Autodesk Inventor part; units mm, degrees
ref_plane "YZ Plane" through (0, 0, 0) normal (1, 0, 0) x (0, 1, 0)
ref_plane "XZ Plane" through (0, 0, 0) normal (0, 1, 0) x (-1, 0, 0)
ref_plane "XY Plane" through (0, 0, 0) normal (0, 0, 1) x (1, 0, 0)
sketch "Sketch1" plane through (0, 0, 0) normal (0, 1, 0) x (-1, 0, 0)
  line L0 (9, 9) -> (-9, 9)
  line L1 (-9, 9) -> (-9, -9)
  line L2 (-9, -9) -> (9, -9)
  line L3 (9, -9) -> (9, 9)
  line L4 (9, 9) -> (-9, -9) construction
  line L5 (-9, 9) -> (9, -9) construction
  line L6 (25, 10) -> (-25, 10)
  line L7 (-25, 10) -> (-25, -10)
  line L8 (-25, -10) -> (25, -10)
  line L9 (25, -10) -> (25, 10)
  line L10 (25, 10) -> (-25, -10) construction
  line L11 (-25, 10) -> (25, -10) construction
  line L12 (25, 0) -> (18, 0)
  line L13 (-25, 0) -> (-18, 0)
  circle A0 centre (18, 0) radius 2.5
  circle A1 centre (-18, 0) radius 2.5
  point P0 (0, 0)
  dimension "d0" = 18
  dimension "d1" = 18
  dimension "d2" = 50
  dimension "d3" = 20
  dimension "d4" = 7
  dimension "d5" = 5
  dimension "d6" = 5
extrude "Extrusion1" add sketch "Sketch1" along normal blind 3 contours L3 L2 L1 L0 | L9 L8 L7 L6
sketch "Sketch2" plane through (0, 3, 0) normal (0, 1, 0) x (1, 0, 0)
  line L0 (-9, 9) -> (9, 9)
  line L1 (9, 9) -> (9, -9)
  line L2 (9, -9) -> (-9, -9)
  line L3 (-9, -9) -> (-9, 9)
  line L4 (-9, 9) -> (9, -9) construction
  line L5 (9, 9) -> (-9, -9) construction
  circle A0 centre (-18, 0) radius 2.5
  circle A1 centre (18, 0) radius 2.5
  line L6 (-25, -10) -> (25, -10)
  line L7 (-25, 10) -> (25, 10)
  line L8 (25, 10) -> (25, -10)
  line L9 (25, -10) -> (-25, -10)
  line L10 (-25, -10) -> (-25, 10)
  line L11 (-25, 10) -> (25, -10) construction
  line L12 (25, 10) -> (-25, -10) construction
  point P0 (0, 0)
  dimension "d9" = 18
  dimension "d10" = 18
extrude "Extrusion2" add sketch "Sketch2" along normal blind 6
sketch "Sketch3" plane through (-25, 0, 10) normal (0, 0, 1) x (1, 0, 0)
  line L0 (34, 3) -> (34, 9)
  line L1 (16, -9) -> (34, -9)
  line L2 (34, -9) -> (34, 9)
  line L3 (34, 9) -> (16, 9)
  line L4 (16, 9) -> (16, -9)
  line L5 (16, -9) -> (34, 9) construction
  line L6 (34, -9) -> (16, 9) construction
  line L7 (16, 0) -> (34, 0)
  point P0 (25, 0)
extrude "Extrusion3" add sketch "Sketch3" along normal blind 10 contours L2 L7 L4 L3 L0
sketch "Sketch4" plane through (0, 9, 0) normal (0, 1, 0) x (1, 0, 0)
  line L0 (-9, -9) -> (9, -9)
  line L1 (0, -9) -> (0, -13)
  line L2 (4, -17) -> (-4, -17)
  line L3 (-4, -17) -> (-4, -9)
  line L4 (-4, -9) -> (4, -9)
  line L5 (4, -9) -> (4, -17)
  line L6 (4, -17) -> (-4, -9) construction
  line L7 (-4, -17) -> (4, -9) construction
  point P0 (0, 0)
  dimension "d15" = 4
  dimension "d16" = 8
extrude "Extrusion4" cut sketch "Sketch4" against normal blind 8
sketch "Sketch5" plane through (0, 3, 0) normal (0, 1, 0) x (1, 0, 0)
  line L0 (-4, -9) -> (4, -9)
  line L1 (0, -9) -> (0, -6)
  line L2 (0, -6) -> (-4, -6)
  line L3 (-4, -6) -> (-4, -9)
  line L4 (-4, -9) -> (0, -9)
  line L5 (0, -9) -> (0, -6)
  line L6 (0, -6) -> (4, -6)
  line L7 (4, -6) -> (4, -9)
  line L8 (4, -9) -> (0, -9)
  line L9 (0, -9) -> (0, -6)
  line L10 (-4, -6) -> (4, -6)
  line L11 (4, -6) -> (4, 0)
  line L12 (4, 0) -> (-4, 0)
  line L13 (-4, 0) -> (-4, -6)
  point P0 (0, 0)
  dimension "d19" = 3
extrude "Extrusion5" cut sketch "Sketch5" against normal blind 2
sketch "Sketch6" plane through (0, 3, 0) normal (0, 1, 0) x (1, 0, 0)
  circle A0 centre (0, 0) radius 2
  dimension "d22" = 4
extrude "Extrusion6" cut sketch "Sketch6" against normal through all
properties part number "gps_holder"
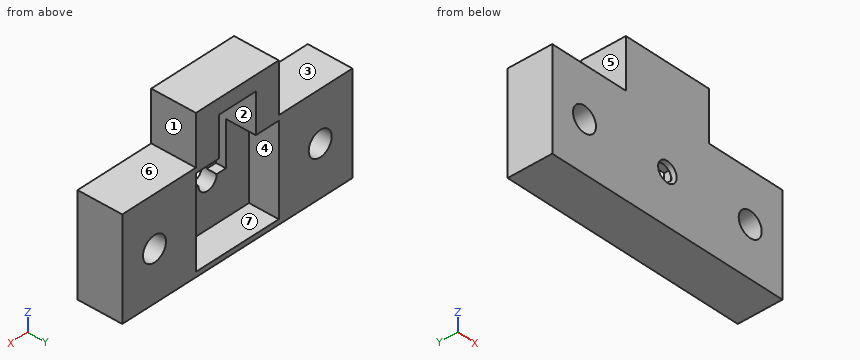
Here's how the part is built. I have some questions about the finished solid (model axes, mm). Face numbers are marked on the shaded views. A direction names the side the tool comes from. Coordinates: 2 decimals unless noted, no trailing zeros. Order: outer loops, then holes, each group sorted by start corner. A loop starts at its lowest first (then second) coordinate and runs counter-clockwise, first axis right, second up. Notation, with made-up numbers: (12, 2) - (44, 2) arc R32 ccw to (44, 36) - close; hole circle Ø6 at (13.25, 0.5). An arc over 180 degrees is marked (long way). Use CSV: the item, a comma, the result in double quotes. Start each with the question number.
1. Suppose I cut it at C-C on x = 7. List the corners of the cut face in (y, z) for me.
2. I'm going to push flat-ended pins straight in: pin 1 (6.5 mm diameter, centred on x = 0.5, z = 8.5, fed in from +Y); pin 2 (1 mm diameter, centred on x = 19, y = 3, fed in from +Z); pin 3 (2.5 mm diameter, centred on y = 6.5, z = 14.5, fed in from -X). Where does each tip first touch, or does it pass through?
3. For the marked faces 5, 6 and 7, which set-ups out of +Z, -Z, +X, -X, +Y, -Y let a thin tool reach every point of the face, with its end or its side?
4. Suppose I cut it at D-D on z = 4.75. List the corners of the cut face in (x, y) for me, then the cut area to 3 significant figures.
5. If we mould it in two halves opening along Z, with no side actions, what happens to the marked faces 1, 2, 3 and 4? For each: +Z half, -Z half, draft (parallel to the pull), parting line (faces both ways), or undercut.
6. Suppose I cut it at A-A on x = 0. List the corners of the cut face in (y, z) for me.
7. Please list where these lines run through material, in increasing order: line 1 (X direction, y = 5.75, z = 0); line 2 (Z direction, x = -18, y = 6); line 3 (Z direction, x = 8, y = 5.5). Write a range as from..to.
8. Suppose I cut it at B-B on y = 5.5. List the corners of the cut face in (x, z) for me.
Output:
1,outline,"(0, -10) - (9, -10) - (9, -9) - (3, -9) - (3, 9) - (9, 9) - (9, 20) - (0, 20) - close"
2,pin 1,"stops at y = 1"
2,pin 2,"stops at z = 10"
2,pin 3,"stops at x = -9"
3,face 5,"+Z, -X, +Y, -Y"
3,face 6,"+Z, +X, +Y, -Y"
3,face 7,"+Y"
4,outline,"(-25, 0) - (25, 0) - (25, 9) - (9, 9) - (9, 3) - (4, 3) - (4, 1) - (-4, 1) - (-4, 3) - (-9, 3) - (-9, 9) - (-25, 9) - close"
4,area,"326 mm2"
5,face 1,"draft"
5,face 2,"undercut"
5,face 3,"+Z half"
5,face 4,"undercut"
6,outline,"(0, -10) - (9, -10) - (9, -9) - (3, -9) - (3, -2) - (0, -2) - close; (0, 2) - (1, 2) - (1, 17) - (9, 17) - (9, 20) - (0, 20) - close"
7,line 1,"x = -25..-20.5, -15.5..-9, 9..15.5, 20.5..25"
7,line 2,"z = -10..-2.5, 2.5..10"
7,line 3,"z = -10..-9, 9..20"
8,outline,"(-25, -10) - (25, -10) - (25, 10) - (9, 10) - (9, 20) - (-9, 20) - (-9, 10) - (-25, 10) - close; hole circle Ø5 at (-18, 0); hole (-9, -9) - (9, -9) - (9, 9) - (4, 9) - (4, 17) - (-4, 17) - (-4, 9) - (-9, 9) - close; hole circle Ø5 at (18, 0)"
